Geometry check sheet. Reference: the model listing, model coordinates, mm. A direction names the side the tool comes from. Give positions to 0.01 mm unless a question says otherwise; leave off trailing zeros. Write each loop counter-clockwise with the first axis right and the second up, starting at its lowest first coordinate (ties: lowest second). Pieces come first, ordered by that corner, then holes. Notation, with made-up numbers: (62.25, 47.5) - (93.25, 47.5) arc R33 cw to (93.25, 85.5) - close; hole circle Ø9 at (49.5, 25). An arc over 180 degrees is marked (long way). Write item = value, one per line. Start each with the question number.
(1) Section check C-C, the plane y = 12.5. Enter the section's corners in (x, z), plus the area to 3 significant figures.
(2) Access from +Z, -Z, +X, -X, +Y, -Y to the whole of each face (thin tool, end or side, straight path). Record for faces 4 (the flat face through (17.5, 14.5, 0)), 5 (the flat face through (18.7, 0, -9.3)), 6 (the cylindrical face through (4.536, 15.014, -9.239)), 7 (the cylindrical face through (33.636, 1.014, -7.715)), 8 (the flat face through (19, 8, -13)).
(3) Depth check by flat-ended pin: pin 1 Ø2.5 at (x, z) = (32, -10) entering from +Y; pin 2 Ø2 at (y, z) = (5, -4.5) entering from -X; pin 3 Ø6 at (x, y) = (18, 5.5) entering from +Z. Enter the tip coordinate at first touch or a pass-through.
(4) Section check D-D, the plane x = 6. Enter the section's corners in (y, z).
(5) Section check A-A, the plane x = 32. Enter the section's corners in (y, z).
(6) Section check B-B, the plane z = -10. Enter the section's corners in (x, y).
(7) Thickness scan on L1, parallel to X at y = 15.6, z = -10; L2, parallel to X at y = 1.2, z = -7.5; L3, parallel to Y at x = 34.5, z = -7. Record the ranges inside material, lowest first.
(8) Draft check along Z on faces 1 (the flat face through (36, 8, -6)), 2 (the cylindrical face through (20.636, 1.014, -7.715)), 3 (the flat face through (19, 8, -15)). Enter one of: pulls with the +Z half, pulls with the -Z half, needs draft (parallel to the pull), parting line crosses it, or undercut.
```python
from build123d import *

# Parameters (mm, degrees)
SKETCH_1_W          = 38
SKETCH_1_H          = 15
EXTRUDE_1_DEPTH     = 16
SKETCH_2_W          = 34
SKETCH_2_H          = 12
CUT_EXTRUDE_1_DEPTH = 13
SKETCH_3_R          = 1.65
CUT_EXTRUDE_2_DEPTH = 2
SKETCH_4_R          = 1.65
CUT_EXTRUDE_3_DEPTH = 10


with BuildPart() as part:
    # 草图1 → 凸台-拉伸1 (new body)
    with BuildSketch(Plane(origin=(0, 0, 0), x_dir=(1, 0, 0), z_dir=(0, 1, 0))):
        with Locations((19, 7.5)):
            Rectangle(SKETCH_1_W, SKETCH_1_H)
    extrude(amount=EXTRUDE_1_DEPTH)

    # 草图2 → 切除-拉伸1 (cut)
    with BuildSketch(Plane.XY):
        with Locations((19, 8)):
            Rectangle(SKETCH_2_W, SKETCH_2_H)
    extrude(amount=-CUT_EXTRUDE_1_DEPTH, mode=Mode.SUBTRACT)

    # 草图3 → 切除-拉伸2 (cut)
    with BuildSketch(Plane(origin=(0, 16, 0), x_dir=(1, 0, 0), z_dir=(0, 1, 0))):
        with Locations(Location((6, 10, 0), (0, 0, 270))):
            Circle(SKETCH_3_R)
        with Locations(Location((32, 10, 0), (0, 0, 90))):
            Circle(SKETCH_3_R)
    extrude(amount=-CUT_EXTRUDE_2_DEPTH, mode=Mode.SUBTRACT)

    # 草图4 → 切除-拉伸3 (cut)
    with BuildSketch(Plane(origin=(0, 2, 0), x_dir=(1, 0, 0), z_dir=(0, 1, 0))):
        with Locations(Location((19, 7.5, 0), (0, 0, 270))):
            Circle(SKETCH_4_R)
        with Locations(Location((32, 7.5, 0), (0, 0, 270))):
            Circle(SKETCH_4_R)
    extrude(amount=-CUT_EXTRUDE_3_DEPTH, mode=Mode.SUBTRACT)


solid = part.part
```
Model answer:
q1.outline = (0, -15) - (38, -15) - (38, 0) - (36, 0) - (36, -13) - (2, -13) - (2, 0) - (0, 0) - close
q1.area = 128 mm²
q2.face_4 = +Z, +X, -X, +Y, -Y
q2.face_5 = +Z, -Z, +X, -X, -Y
q2.face_6 = +Y
q2.face_7 = -Y
q2.face_8 = +Z
q3.pin_1 = 2
q3.pin_2 = 0
q3.pin_3 = -13
q4.outline = (0, -15) - (16, -15) - (16, -11.65) - (14, -11.65) - (14, -13) - (2, -13) - (2, 0) - (0, 0) - close; (14, -8.35) - (16, -8.35) - (16, 0) - (14, 0) - close
q5.outline = (0, -15) - (16, -15) - (16, -11.65) - (14, -11.65) - (14, -13) - (2, -13) - (2, -9.15) - (0, -9.15) - close; (0, -5.85) - (2, -5.85) - (2, 0) - (0, 0) - close; (14, -8.35) - (16, -8.35) - (16, 0) - (14, 0) - close
q6.outline = (0, 0) - (38, 0) - (38, 16) - (33.65, 16) - (33.65, 14) - (36, 14) - (36, 2) - (2, 2) - (2, 14) - (4.35, 14) - (4.35, 16) - (0, 16) - close; (7.65, 14) - (30.35, 14) - (30.35, 16) - (7.65, 16) - close
q7.L1 = 0 to 4.35, 7.65 to 30.35, 33.65 to 38
q7.L2 = 0 to 17.35, 20.65 to 30.35, 33.65 to 38
q7.L3 = 0 to 2, 14 to 16
q8.face_1 = needs draft
q8.face_2 = undercut
q8.face_3 = pulls with the -Z half
